Verification items for the finished model (mm, model axes). Round coordinates to 2 decimals unless told otherwise and drop trailing zeros. Write each loop counter-clockwise with the first axis right and the second up, starting at its lowest first coordinate (ties: lowest second). Pieces come first, ordered by that corner, then holes. Notation, with made-up numbers: (8, 22) - (17, 22) arc R19 ccw to (17, 39) - close; hole circle Ø3 at (-16.5, -5.5). An arc over 180 degrees is marked (long way). Answer as a JSON object with one key per item and string values.
```python
from build123d import *

# Parameters (mm, degrees)
F0_W     = 30
F0_H     = 30
F1_DEPTH = 10
F3_DEPTH = 50
F5_D     = 5
F6_R     = 2
F7_R     = 1


with BuildPart() as f1:
    # F0 (on Top) → F1 (new body)
    with BuildSketch(Plane.XY):
        Rectangle(F0_W, F0_H)
    extrude(amount=F1_DEPTH)

    # F2 (on face) → F3 (cut)
    with BuildSketch(Plane.XZ.offset(15)):
        with BuildLine():
            Line((15, 10), (-15, 10))
            ThreePointArc((-15, 10), (0, 6.869318), (15, 10))
        make_face()
    extrude(amount=-F3_DEPTH, mode=Mode.SUBTRACT)

    # F5 (through all)
    with Locations(Plane(origin=(0, 0, 0), x_dir=(1, 0, 0), z_dir=(0, 0, -1))):
        with Locations((0, 0)):
            Hole(F5_D / 2)

    # F6
    f6_edges = [f1.edges().sort_by_distance(p)[0] for p in [
        (-15, -15, 5),
        (15, -15, 5),
        (15, 15, 5),
        (-15, 15, 5),
    ]]
    fillet(f6_edges, radius=F6_R)

    # F7
    f7_edges = [f1.edges().sort_by_distance(p)[0] for p in [
        (-15, 0, 0),
    ]]
    fillet(f7_edges, radius=F7_R)


solid = f1.part
```
Q1. Material ranges on line 1 along Y through (x, z) = (0, 5); line 2 along Y through (x, z) = (1.5, 3.25); line 3 along Z through (x, y) = (13, 2), recorded low to high. Write a range as [from, to].
Geometry check:
{"line 1": "y = [-15, -2.5], [2.5, 15]", "line 2": "y = [-15, -2], [2, 15]", "line 3": "z = [0, 9.19]"}
Q2. Section check D-D, the plane y = -10.5. Record the cut outline in (x, z), then the cut area to 3 significant figures.
Geometry check:
{"outline": "(-15, 1) arc R1 ccw to (-14, 0) - (14, 0) arc R1 ccw to (15, 1) - (15, 10) arc R37.5 cw to (-15, 10) - close", "area": "236 mm2"}
Q3. Release check for a two-part mould opening along Y. For faces 1 (the cylindrical face through (14.4, 14.43, 5.56)), 2 (the flat face through (-15, 0, 5)), 3 (the cylindrical face through (0.54, 2.44, 3.53)) record: released by +Y, released by -Y, zero draft, split by the parting line, or undercut.
Geometry check:
{"face 1": "released by +Y", "face 2": "zero draft", "face 3": "undercut"}
Q4. Section check B-B, the plane x = 0. Record the cut outline in (y, z).
Geometry check:
{"outline": "(-15, 1) arc R1 ccw to (-14, 0) - (-2.5, 0) - (-2.5, 6.87) - (-15, 6.87) - close; (2.5, 0) - (14, 0) arc R1 ccw to (15, 1) - (15, 6.87) - (2.5, 6.87) - close"}
Q5. Gauge pin test, flat end, axial feed: P1, Ø8, axis at x = -7, y = -5.5, coming from the +Z side. Record the tip position at first contact, or that the pin passes through.
Geometry check:
{"P1": "stops at z = 8.52"}
Q6. Section check C-C, the plane z = 8. Record the cut outline in (x, y).
Geometry check:
{"outline": "(-15, -13) arc R2 ccw to (-13, -15) - (-9.14, -15) - (-9.14, 15) - (-13, 15) arc R2 ccw to (-15, 13) - close; (9.14, -15) - (13, -15) arc R2 ccw to (15, -13) - (15, 13) arc R2 ccw to (13, 15) - (9.14, 15) - close"}
Q7. Section check A-A, the plane y = 0. Record the cut outline in (x, z).
Geometry check:
{"outline": "(-15, 1) arc R1 ccw to (-14, 0) - (-2.5, 0) - (-2.5, 6.95) arc R37.5 cw to (-15, 10) - close; (2.5, 0) - (14, 0) arc R1 ccw to (15, 1) - (15, 10) arc R37.5 cw to (2.5, 6.95) - close"}
